```python
from build123d import *

# Parameters (mm, degrees)
F0_W        = 17
F0_H        = 2
F0_H_2      = 15
F1_DEPTH    = 8
F2_R        = 5
F3_T1_DEPTH = 8
F3_T3_DEPTH = 18.3525106995
F3_T5_DEPTH = 21.4805273161
F4_R        = 1
F5_R        = 2.99999


# Not quite as in the source:
# - a fillet or chamfer that OpenCascade refuses, or shapes differently, is made with other operations: its cross-section is extruded or revolved along the edge and cut away or added
# - a fillet or chamfer is up to 0.001 mm smaller than in the source, because OpenCascade refuses the exact size


with BuildPart() as f1:
    # F0 (on Top) → F1 (new body)
    with BuildSketch(Plane.XY):
        with BuildLine():
            ThreePointArc((2.7332443879, -3.5748251868), (-4.4992296638, -0.0832612306), (2.5991092476, 3.6735039294))
            Line((2.5991092476, 3.6735039294), (5.3624032747, 3.6735039294))
            ThreePointArc((5.3624032747, 3.6735039294), (-3.1508257353, 5.6852701946), (-5.9573484034, -2.6))
            Line((-5.9573484034, -2.6), (-15.4573484034, -2.6))
            Line((-15.4573484034, -2.6), (-15.4573484034, 13.4))
            Line((-15.4573484034, 13.4), (-15.4573484034, 17.4032363431))
            Line((-15.4573484034, 17.4032363431), (-36.4629774356, 17.4032363431))
            Line((-36.4629774356, 17.4032363431), (-36.4629774356, 11.4032363431))
            Line((-36.4629774356, 11.4032363431), (-36.4629774356, -9.5967636569))
            Line((-36.4629774356, -9.5967636569), (-15.4629774356, -9.5967636569))
            Line((-15.4629774356, -9.5967636569), (-15.4629774356, -5.5967636569))
            Line((-15.4629774356, -5.5967636569), (-5.3631004506, -5.5967636569))
            ThreePointArc((-5.3631004506, -5.5967636569), (1.2632530504, -7.6479279289), (6.8780254985, -3.5748251868))
            Line((6.8780254985, -3.5748251868), (2.7332443879, -3.5748251868))
        make_face()
        with Locations((-25.9629774356, -6.6)):
            Rectangle(F0_W, F0_H, mode=Mode.SUBTRACT)
        with Locations((-25.9573484034, 3.9)):
            Rectangle(F0_W, F0_H_2, mode=Mode.SUBTRACT)
        with Locations((-25.9573484034, 14.4032363431)):
            Rectangle(F0_W, F0_H, mode=Mode.SUBTRACT)
    extrude(amount=F1_DEPTH)

    # F2
    f2_edges = [f1.edges().sort_by_distance(p)[0] for p in [
        (-5.957348, -2.6, 4),
        (-5.3631, -5.596764, 4),
    ]]
    fillet(f2_edges, radius=F2_R)

    # F3: chamfer of 1 on 6 edges, made by hand

    # F3_s2 → F3_t1 (join)
    with BuildSketch(Plane.XY):
        Polygon((-34.4573484034, -2.6), (-33.4573484034, -3.6), (-34.4573484034, -3.6), align=None)
        Polygon((-34.4573484034, 10.4), (-33.4573484034, 11.4), (-34.4573484034, 11.4), align=None)
        Polygon((-18.4573484034, 11.4), (-17.4573484034, 10.4), (-17.4573484034, 11.4), align=None)
        Polygon((-17.4573484034, -2.6), (-18.4573484034, -3.6), (-17.4573484034, -3.6), align=None)
    extrude(amount=F3_T1_DEPTH)

    # F3_s4 → F3_t3 (cut)
    with BuildSketch(Plane.XY.offset(-5.1762553498)):
        with BuildLine():
            Line((5.7007617196, -5.2524209363), (4.9653271539, -3.5748251868))
            Line((4.9653271539, -3.5748251868), (6.8780254985, -3.5748251868))
            ThreePointArc((6.8780254985, -3.5748251868), (6.3390727508, -4.4612516781), (5.7007617196, -5.2524209363))
        make_face()
    extrude(amount=F3_T3_DEPTH, mode=Mode.SUBTRACT)

    # F3_s6 → F3_t5 (cut)
    with BuildSketch(Plane.XY.offset(-6.740263658)):
        with BuildLine():
            Line((2.8997174039, 3.6735039294), (3.42693875, 5.5232319165))
            ThreePointArc((3.42693875, 5.5232319165), (4.4840607821, 4.7056560544), (5.3624032747, 3.6735039294))
            Line((5.3624032747, 3.6735039294), (2.8997174039, 3.6735039294))
        make_face()
    extrude(amount=F3_T5_DEPTH, mode=Mode.SUBTRACT)

    # F4
    f4_edges = [f1.edges().sort_by_distance(p)[0] for p in [
        (-15.462977, -9.596764, 4),
        (-36.462977, 17.403236, 4),
        (-15.457348, 17.403236, 4),
        (-36.462977, -9.596764, 4),
    ]]
    fillet(f4_edges, radius=F4_R)

    # F5 (radius 3 in the source; OpenCascade refuses exactly that, so slightly less here)
    f5_edges = [f1.edges().sort_by_distance(p)[0] for p in [
        (-15.457348, -2.6, 4),
        (-15.462977, -5.596764, 4),
    ]]
    fillet(f5_edges, radius=F5_R)


solid = f1.part
```
Can you work these out from the model? Positions are in its coordinate system, mm. A direction names the side the tool comes from. Give positions to 0.01 mm unless a question says otherwise; leave off trailing zeros. Loops run counter-clockwise (first coordinate to the right, second up) from the corner with the lowest first, then second, coordinate; pieces in that order, holes last. Notation, with made-up numbers: M 88,75 L 124,75 A34 ccw 124,113 Z; hole C 14.5,76.5 d1. An arc over 180 degrees is marked long. One line per item, written item: value.
(1) Suppose I cut it at A-A on x = -31. List the corners of the cut face in (y, z) for me, plus the area to 3 significant figures.
Returned:
outline: M -9.6,0 L -7.6,0 L -7.6,8 L -9.6,8 Z; M -5.6,0 L -3.6,0 L -3.6,8 L -5.6,8 Z; M 11.4,0 L 13.4,0 L 13.4,8 L 11.4,8 Z; M 15.4,0 L 17.4,0 L 17.4,8 L 15.4,8 Z
area: 64.0 mm^2
(2) Suppose I cut it at D-D on z = 4.5. Count the separate pieces of the cut face and the enclosed holes in it, plus the area to 3 significant figures.
Returned:
separate pieces: 1
enclosed holes: 3
area: 350 mm^2
(3) Suppose I cut it at B-B on y = 9.5. List the corners of the cut face in (x, z) for me.
Returned:
outline: M -36.46,0 L -34.46,0 L -34.46,8 L -36.46,8 Z; M -17.46,0 L -15.46,0 L -15.46,8 L -17.46,8 Z
(4) Will these pins go through, and if not, where does the flat tip stop? pin 1 (4 mm diameter, centred on y = 12, z = 2.5, fed in from +X); pin 2 (2 mm diameter, centred on y = -7, z = 5, fed in from +X); pin 3 (4.5 mm diameter, centred on x = -10, z = 4.5, fed in from -Y).
Returned:
pin 1: x = -15.46
pin 2: x = 4.91
pin 3: y = -5.6
(5) Suppose I cut it at C-C on x = 0. List the corners of the cut face in (y, z) for me.
Returned:
outline: M -7.75,0 L -4.5,0 L -4.5,8 L -7.75,8 Z; M 4.5,0 L 6.5,0 L 6.5,8 L 4.5,8 Z
(6) We'd pull the mould along X, two halves only. Please class faces 1 (the face through (3.16, 4.59, 3.94)), 2 (the face through (-17.457, 4, 4)), 3 (the face through (-17, 2, 0)), 4 (the face through (-17.95, -3.09, 3.94)): released by +X, released by -X, zero draft, split by the parting line, or undercut.
Returned:
face 1: released by +X
face 2: undercut
face 3: zero draft
face 4: undercut
(7) Which directions (+Z, -Z, +X, -X, +Y, -Y) give clear straight access to the entire face, cutting with the end or side of a thin tool? Please do faces 5 (the face through (-10, -5.597, 4)), 6 (the face through (-26, -7.6, 4)), 7 (the face through (-15.457, 8, 4)).
Returned:
face 5: +Z, -Z, -Y
face 6: +Z, -Z
face 7: +Z, -Z, +Y
(8) I need wall thicknesses on line 1 (Y direction, x = -33, z = 4.25); line 2 (X direction, y = 15, z = 6); line 3 (Y direction, x = 0, z = 5.5). Which ranges of each line are inside material? Lowest first, please.
Returned:
line 1: -9.6 to -7.6, -5.6 to -3.6, 11.4 to 13.4, 15.4 to 17.4
line 2: -36.46 to -34.46, -17.46 to -15.46
line 3: -7.75 to -4.5, 4.5 to 6.5
